Check sheet for the modelled part. Datum: model origin and axes. Units: mm. A direction names the side the tool comes from. Round coordinates to 2 decimals unless told otherwise and drop trailing zeros. Order: outer loops, then holes, each group sorted by start corner. A loop starts at its lowest first (then second) coordinate and runs counter-clockwise, first axis right, second up.
Q1. Cross-section at A-A on y = -12. Record the cut outline in (x, z).
Q2. Cross-section at C-C on z = 17.5. Record the cut outline in (x, y).
Q3. Depth check by flat-ended pin: P1, Ø23, axis at x = -51.53, z = 50.8, coming from the +Y side; P2, Ø20.5, axis at y = -40.5, z = 33, coming from the +X side; P3, Ø1.5, axis at y = -35, z = 55.5, coming from the -X side; P4, Ø5, axis at y = -9.5, z = 67.5, coming from the -X side. Enter the tip coordinate at first touch or a pass-through.
Q4. Cross-section at D-D on x = 9. Record the cut outline in (y, z).
Q5. Cross-section at B-B on x = -58. Record the cut outline in (y, z), then the cut area to 3 significant figures.
Q6. Mould release check, pull along X, two halves, no side actions. Record for faces 3 (the flat face through (-45, -50.8, 32)), 4 (the cylindrical face through (47.121, -48.002, 9.312)), 5 (the flat face through (-76.929, -25, 27)): +X half, -X half, draft (parallel to the pull), parting line (faces both ways), or undercut.
Q7. Scan lines: probe 1 along Z at (x, y) = (-24.5, -46.5); probe 2 along X at (y, z) = (-29.5, 29); probe 3 along Z at (x, y) = (-47.5, -10). Record each from-to range of solid material in increasing order.
Q8. Set-up check for faces 1 (the flat face through (-28, 0, 32)), 2 (the flat face through (13, -38, 15.17)): record each of +Z, -Z, +X, -X, +Y, -Y from which the full face is reachable in a straight line by a thin tool's end or side.
from build123d import *
from build123d import SkipClean  # not in build123d's __all__

# Parameters (mm, degrees)
F1_DEPTH = 25.4
F2_R     = 12.7
F3_DEPTH = 25.4
F4_R     = 9.8113639175


with BuildPart() as f1:
    # F0 (on Front) → F1 (new body)
    with BuildSketch(Plane.XZ):
        with BuildLine():
            ThreePointArc((-37.8463725496, 72.1998437426), (-63.7276630417, 73.0788204047), (-76.9287220478, 50.8))
            Line((-76.9287220478, 50.8), (-76.9287220478, 3.2882173546))
            Line((-76.9287220478, 3.2882173546), (50.0712779522, 3.2882173546))
            Line((50.0712779522, 3.2882173546), (50.0712779522, 15.9882173546))
            Line((50.0712779522, 15.9882173546), (-37.8463725496, 72.1998437426))
        make_face()
        with BuildLine():
            ThreePointArc((-64.2287220478, 50.8), (-51.5287220478, 63.5), (-38.8287220478, 50.8))
            ThreePointArc((-38.8287220478, 50.8), (-51.5287220478, 38.1), (-64.2287220478, 50.8))
        make_face(mode=Mode.SUBTRACT)
    extrude(amount=F1_DEPTH)

    # F2 (on face) → F3 (join)
    with BuildSketch(Plane.XZ.offset(25.4)):
        with BuildLine():
            Line((-26.1287220478, 15.9882173546), (-26.1287220478, 50.8))
            ThreePointArc((-26.1287220478, 50.8), (-29.2499016431, 62.9989409939), (-37.8463725496, 72.1998437426))
            ThreePointArc((-37.8463725496, 72.1998437426), (-63.7276630417, 73.0788204047), (-76.9287220478, 50.8))
            Line((-76.9287220478, 50.8), (-76.9287220478, 15.1695013046))
            Line((-76.9287220478, 15.1695013046), (-76.9287220478, 3.2882173546))
            Line((-76.9287220478, 3.2882173546), (50.0712779522, 3.2882173546))
            Line((50.0712779522, 3.2882173546), (50.0712779522, 15.1695013046))
            Line((50.0712779522, 15.1695013046), (-26.1287220478, 15.1695013046))
            Line((-26.1287220478, 15.1695013046), (-26.1287220478, 15.9882173546))
        make_face()
        with Locations((-51.5287220478, 50.8)):
            Circle(F2_R, mode=Mode.SUBTRACT)
    with SkipClean():  # cleaning this boolean's faces spoils the solid; the shape is the same uncleaned
        extrude(amount=F3_DEPTH)

    # F4
    f4_edges = [f1.edges().sort_by_distance(p)[0] for p in [
        (50.071278, -50.8, 9.228859),
    ]]
    fillet(f4_edges, radius=F4_R)


solid = f1.part
Results found:
1. outline: (-76.93, 3.29) - (50.07, 3.29) - (50.07, 15.99) - (-37.85, 72.2) arc R25.4 ccw to (-76.93, 50.8) - close; hole circle Ø25.4 at (-51.53, 50.8)
2. outline: (-76.93, -50.8) - (-26.13, -50.8) - (-26.13, -25.4) - (47.71, -25.4) - (47.71, 0) - (-76.93, 0) - close
3. P1: passes through
3. P2: stops at x = -26.13
3. P3: stops at x = -76.62
3. P4: stops at x = -72.59
4. outline: (-50.8, 3.29) - (0, 3.29) - (0, 42.25) - (-25.4, 42.25) - (-25.4, 15.17) - (-50.8, 15.17) - close
5. outline: (-50.8, 3.29) - (0, 3.29) - (0, 39.87) - (-50.8, 39.87) - close; (-50.8, 61.73) - (0, 61.73) - (0, 75.36) - (-50.8, 75.36) - close
5. area: 2,550 mm2
6. face 3: draft
6. face 4: +X half
6. face 5: -X half
7. probe 1: z = 3.29 to 15.17
7. probe 2: x = -76.93 to -26.13
7. probe 3: z = 3.29 to 38.76, 62.84 to 75.88
8. face 1: +Z, -Z, +X, -X, +Y
8. face 2: +Z, +X, -Y
